Geometry: final body of the model. Coordinates: model frame, mm. Face numbers are marked on the shaded views. A direction names the side the tool comes from. Round coordinates to 2 decimals unless told otherwise and drop trailing zeros. Write each loop counter-clockwise with the first axis right and the second up, starting at its lowest first coordinate (ties: lowest second). Pieces come first, ordered by that corner, then holes. Notation, with made-up numbers: M 10,19 L 68,19 A8 ccw 68,23 Z; hole C 45.25,-31 d11. An arc over 180 degrees is marked long. Use one line per item in the form item = value. Start each with the question number.
Item 1: Section query D-D (y = -1.5). Return loops of the section in (x, z), and give its area (3 significant figures).
Item 2: Section query B-B (y = -5). Return loops of the section in (x, z).
Item 3: Section query C-C (z = 18.25). Return loops of the section in (x, y), and give its area (3 significant figures).
Item 4: Pin query (flat end, axial travel): pin 1 Ø1 at (x, z) = (1.5, 8) entering from +Y; pin 2 Ø2 at (x, z) = (1.5, 2.5) entering from -Y; pin 3 Ø8 at (x, z) = (6, 15.5) entering from -Y; pin 4 Ø2 at (y, z) = (-2, 17.5) entering from -X. Return the tip coordinate at first contact, or that it passes through.
Item 5: Reachability of the marked faces 4, 5, 6 and 7 from +Z, -Z, +X, -X, +Y, -Y: full face, straight path, thin tool, end or side. Return the list, or none.
Item 6: Pull-direction query (Y, two-part tool) for the marked faces 1, 2 and 3; classes: pulls with the +Y half, pulls with the -Y half, needs draft (parallel to the pull), parting line crosses it, or undercut.
Item 7: Ray query, probe 1 along Z at (x, y) = (8.1, 0); probe 2 along Z at (x, y) = (4.5, -2.75); probe 3 along X at (y, z) = (-8.25, 4.5). Return the intervals inside material, ascending.
Item 8: Section query A-A (z = 10). Return loops of the section in (x, y), and give its area (3 significant figures).
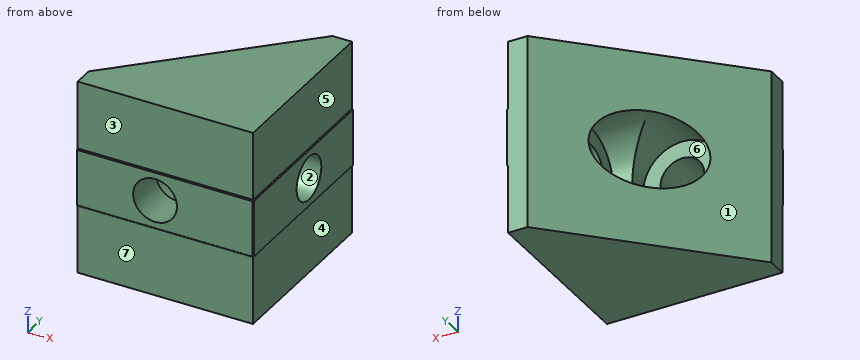
from build123d import *

# Parameters (mm, degrees)
SKETCH_W        = 20
SKETCH_H        = 20
PAD_DEPTH       = 20
PAD001_DEPTH    = 20
PAD002_DEPTH    = 20
SKETCH004_R     = 2.25
POCKET001_DEPTH = 20.1
SKETCH005_R     = 4
POCKET002_DEPTH = 16
SKETCH006_R     = 2.25
POCKET003_DEPTH = 20.1
SKETCH007_R     = 4
POCKET004_DEPTH = 16
POCKET_DEPTH    = 20


with BuildPart() as part:
    # Sketch → Pad (new body)
    with BuildSketch(Plane.XY):
        Rectangle(SKETCH_W, SKETCH_H)
    extrude(amount=PAD_DEPTH)

    # Sketch001 (on DatumPlane) → Pad001 (join)
    with BuildSketch(Plane.XZ.offset(10)):
        Polygon((10, 13), (10.1, 12.9), (10.1, 7.1), (10, 7), align=None)
    extrude(amount=-PAD001_DEPTH)

    # Sketch002 (on DatumPlane) → Pad002 (join)
    with BuildSketch(Plane.YZ.offset(10)):
        Polygon((-10, 13), (-10, 7), (-10.1, 7.1), (-10.1, 12.9), align=None)
    extrude(amount=-PAD002_DEPTH)

    # Sketch004 (on DatumPlane) → Pocket001 (cut)
    with BuildSketch(Plane(origin=(-10, 0, 0), x_dir=(0, -1, 0), z_dir=(-1, 0, 0))):
        with Locations((20, 10)):
            Circle(SKETCH004_R)
        with Locations((0, 10)):
            Circle(SKETCH004_R)
    extrude(amount=-POCKET001_DEPTH, mode=Mode.SUBTRACT)

    # Sketch005 (on DatumPlane) → Pocket002 (cut)
    with BuildSketch(Plane(origin=(-10, 0, 0), x_dir=(0, -1, 0), z_dir=(-1, 0, 0))):
        with Locations((20, 10)):
            Circle(SKETCH005_R)
        with Locations((0, 10)):
            Circle(SKETCH005_R)
    extrude(amount=-POCKET002_DEPTH, mode=Mode.SUBTRACT)

    # Sketch006 (on DatumPlane) → Pocket003 (cut)
    with BuildSketch(Plane(origin=(0, 10, 0), x_dir=(-1, 0, 0), z_dir=(0, 1, 0))):
        with Locations((0, 10)):
            Circle(SKETCH006_R)
        with Locations((20, 10)):
            Circle(SKETCH006_R)
    extrude(amount=-POCKET003_DEPTH, mode=Mode.SUBTRACT)

    # Sketch007 (on DatumPlane) → Pocket004 (cut)
    with BuildSketch(Plane(origin=(0, 10, 0), x_dir=(-1, 0, 0), z_dir=(0, 1, 0))):
        with Locations((0, 10)):
            Circle(SKETCH007_R)
        with Locations((20, 10)):
            Circle(SKETCH007_R)
    extrude(amount=-POCKET004_DEPTH, mode=Mode.SUBTRACT)

    # Sketch008 (on DatumPlane) → Pocket (cut)
    with BuildSketch(Plane.XY.offset(20)):
        Polygon((10.1, 10.1), (-10.1, 10.1), (-10.1, -10.1), (-8, -10.1), (-8, -8), (8, 8), (10.1, 8), align=None)
    extrude(amount=-POCKET_DEPTH, mode=Mode.SUBTRACT)


solid = part.part
Working result:
q1.outline = M -1.5,0 L 10,0 L 10,7 L 10.1,7.1 L 10.1,8.32 L 6,8.32 L 6,6.29 L 1.5,6.29 A4 cw -1.5,6.29 Z; M -1.5,13.71 A4 cw 1.5,13.71 L 6,13.71 L 6,11.68 L 10.1,11.68 L 10.1,12.9 L 10,13 L 10,20 L -1.5,20 Z
q1.area = 160 mm²
q2.outline = M -5,0 L 10,0 L 10,7 L 10.1,7.1 L 10.1,12.9 L 10,13 L 10,20 L -5,20 Z; hole C 0,10 d8
q3.outline = M -8,-10 L 10,-10 L 10,8 L 8,8 L -8,-8 Z
q3.area = 196 mm²
q4.pin_1 = -6
q4.pin_2 = -10
q4.pin_3 = -10.1
q4.pin_4 = -3
q5.face_4 = -Z, +X, +Y, -Y
q5.face_5 = +Z, +X, +Y, -Y
q5.face_6 = +Y
q5.face_7 = -Z, +X, -X, -Y
q6.face_1 = pulls with the +Y half
q6.face_2 = undercut
q6.face_3 = pulls with the -Y half
q7.probe_1 = 0 to 7.75, 12.25 to 20
q7.probe_2 = 0 to 7.1, 12.9 to 20
q7.probe_3 = -8 to 10
q8.outline = M -8,-10.1 L -2.25,-10.1 L -2.25,-6 L -4,-6 L -4,-4 L -8,-8 Z; M 2.25,-10.1 L 10,-10.1 L 10,-10 L 10.1,-10 L 10.1,-2.25 L 6,-2.25 L 6,-4 L 4,-4 L 4,-6 L 2.25,-6 Z; M 4,4 L 6,4 L 6,2.25 L 10.1,2.25 L 10.1,8 L 8,8 Z
q8.area = 98.7 mm²
